The model under review builds one solid part; all positions refer to its coordinate system, in mm. A direction names the side the tool comes from. Give positions to 0.01 mm unless a question says otherwise; leave off trailing zeros. Order: outer loops, then holes, each group sorted by start corner. A loop starts at its lowest first (then second) coordinate and runs counter-clockwise, first axis right, second up. Notation, with made-up numbers: M 39.25,-15.5 L 51.25,-15.5 A18 ccw 51.25,16.5 Z; hole C 59,-2 d8. An arc over 180 degrees is marked long. One line per question, with ' | ' between items. Start each with the question number.
1. We need section D-D on y = 43.5. Write out the cut boundary in (x, z), then the cut area to 3 significant figures.
2. We need section B-B on y = 30. Write out the cut boundary in (x, z), then the cut area to 3 significant figures.
3. The part is to be moulded in two halves that separate along Z. For faces 1 (the face through (49, 38, 53.301)), 2 (the face through (49, 31, 23)), 3 (the face through (60, 1, 12)), say which applies: +Z half, -Z half, draft (parallel to the pull), parting line (faces both ways), or undercut.
4. Insertion check: P1, Ø2, axis at y = 30, z = 33.5, coming from the -X side; P2, Ø1.6, axis at y = 1, z = 12.5, coming from the -X side; P3, Ø1, axis at y = 1, z = 12.5, coming from the +X side; P4, Ø9, axis at x = 49, y = 3, coming from the +Z side. Each pin has a flat end and moves straight along its axis. Give the tip position at first contact, or say it passes through.
5. We need section C-C on x = 50. Write out the cut boundary in (y, z).
6. For faces 4 (the face through (49, 36, 28)), 5 (the face through (49.3, 23.605, 23.172)), 6 (the face through (40, 1, 12)), 7 (the face through (50, 1, 15)), list the 3-axis set-ups (+Z, -Z, +X, -X, +Y, -Y) from which the entire face can be reached by the end or side of a thin tool; tool diameter is ignored.
7. Wall thickness on L1, parallel to Y at x = 42, z = 13.5; L2, parallel to Z at x = 39.5, y = 38.5; L3, parallel to Y at x = 38.5, z = 13: over which ranges is each line inside the solid? List them lowest first.
8. We need section A-A on z = 22. Write out the cut boundary in (x, y).
Autodesk Fusion 360 part; units mm, degrees
sketch "Sketch1" plane through (0, 0, 0) normal (0, 0, 1) x (1, 0, 0)
  line L0 (0, 0) -> (0, 50)
  line L1 (0, 50) -> (100, 50)
  line L2 (100, 50) -> (100, 0)
  line L3 (100, 0) -> (0, 0)
  dimension "d2" = 50
  dimension "d3" = 100
  dimension "d4" = 50
extrude "Extrude1" add sketch "Sketch1" along normal blind 10
sketch "Sketch2" plane through (0, 0, 0) normal (1, 0, 0) x (0, 1, 0)
  line L0 (0, 10) -> (11, 10)
  line L1 (11, 10) -> (36, 53.3013) construction
  line L2 (11, 10) -> (36, 53.3013)
  line L3 (36, 53.3013) -> (41, 53.3013)
  line L4 (41, 53.3013) -> (16, 10)
  line L5 (16, 10) -> (11, 10)
  line L6 (41, 53.3013) -> (36, 44.641)
  line L7 (36, 44.641) -> (36, 10)
  line L8 (36, 10) -> (31, 10)
  line L9 (31, 10) -> (31, 35.9808)
  dimension "d7" = 11
  dimension "d10" = 50
  dimension "d11" = 5
  dimension "d12" = 10
  dimension "d13" = 5
extrude "Extrude2" add sketch "Sketch2" along normal blind 100
sketch "Sketch3" plane through (0, 0, 10) normal (0, 0, 1) x (-1, 0, 0)
  line L0 (-100, -11) -> (0, -11)
  line L1 (0, -11) -> (0, 0)
  line L2 (0, 0) -> (-100, 0)
  line L3 (-100, 0) -> (-100, -11)
  line L4 (-50, 0) -> (-60, 0)
  line L5 (-50, 0) -> (-40, 0)
  line L6 (-60, 0) -> (-60, -2)
  line L7 (-60, -2) -> (-40, -2)
  line L8 (-40, -2) -> (-40, 0)
  dimension "d16" = 10
  dimension "d17" = 10
  dimension "d18" = 2
extrude "Extrude3" add sketch "Sketch3" along normal blind 5 contours L2 L4 L5 L6 L7 L8
Entries:
1) outline: M 0,0 L 100,0 L 100,10 L 0,10 Z | area: 1,000 mm^2
2) outline: M 0,0 L 100,0 L 100,10 L 0,10 Z; M 0,34.25 L 100,34.25 L 100,42.91 L 0,42.91 Z | area: 1,870 mm^2
3) face 1: +Z half | face 2: undercut | face 3: draft
4) P1: stops at x = 0 | P2: stops at x = 40 | P3: stops at x = 60 | P4: stops at z = 15
5) outline: M 0,0 L 50,0 L 50,10 L 36,10 L 36,44.64 L 41,53.3 L 36,53.3 L 11,10 L 2,10 L 2,15 L 0,15 Z; hole M 16,10 L 31,10 L 31,35.98 Z
6) face 4: +X, -X, +Y | face 5: +X, -X | face 6: +Z, -X, -Y | face 7: +Z, +X, -X, -Y
7) L1: y = 0 to 2, 13.02 to 18.02, 31 to 36 | L2: z = 0 to 10, 48.97 to 53.3 | L3: y = 12.73 to 17.73, 31 to 36
8) outline: M 0,17.93 L 100,17.93 L 100,22.93 L 0,22.93 Z; M 0,31 L 100,31 L 100,36 L 0,36 Z
